Input: part model. Units: mm. Frame: model coordinates. Round coordinates to 2 decimals unless told otherwise and drop trailing zeros. Loops run counter-clockwise (first coordinate to the right, second up) from the corner with the lowest first, then second, coordinate; pieces in that order, holes last.
(1) First-contact query: pin 1 Ø2.5 at (x, y) = (12, -35) entering from +Z. Flat tip, straight axial feed; report the tip coordinate or a pass-through.
(2) Line query: line 1 (X direction, y = -12, z = 1.5); line 2 (Y direction, x = 31, z = 3); line 3 (X direction, y = -35, z = 3.5). Output: solid intervals per line, ascending.
(3) Cut plane D-D, the plane z = 3.25. Give the number of separate pieces and of enclosed holes in the cut face, and give its area (3 significant figures).
(4) Cut plane A-A, the plane x = 77. Output: boundary loops of the cut face in (y, z).
(5) Cut plane C-C, the plane x = 5. Output: boundary loops of the cut face in (y, z), and give its area (3 significant figures).
(6) Cut plane B-B, the plane y = -20.5. Output: boundary loops of the cut face in (x, z), and give its area (3 significant figures).
from build123d import *

# Parameters (mm, degrees)
F0_W     = 100
F0_H     = 40
F1_DEPTH = 5
F2_R     = 2.25
F3_DEPTH = 18.9
F5_DEPTH = 0.5
F7_DEPTH = 5


with BuildPart() as f1:
    # F0 (on Top) → F1 (new body)
    with BuildSketch(Plane.XY):
        with Locations((50, -20)):
            Rectangle(F0_W, F0_H)
    extrude(amount=F1_DEPTH)

    # F2 (on Top) → F3 (cut)
    with BuildSketch(Plane.XY):
        with Locations((12, -35)):
            Circle(F2_R)
        with Locations((31, -35)):
            Circle(F2_R)
        with Locations((50, -35)):
            Circle(F2_R)
        with Locations((69, -35)):
            Circle(F2_R)
        with Locations((88, -35)):
            Circle(F2_R)
        with Locations((95, -28)):
            Circle(F2_R)
        with Locations((95, -12)):
            Circle(F2_R)
        with Locations((88, -5)):
            Circle(F2_R)
        with Locations((69, -5)):
            Circle(F2_R)
        with Locations((50, -5)):
            Circle(F2_R)
        with Locations((31, -5)):
            Circle(F2_R)
        with Locations((12, -5)):
            Circle(F2_R)
        with Locations((5, -12)):
            Circle(F2_R)
        with Locations((5, -28)):
            Circle(F2_R)
    extrude(amount=F3_DEPTH, mode=Mode.SUBTRACT)

    # F4 (on face) → F5 (cut)
    with BuildSketch(Plane(origin=(0, 0, 0), x_dir=(1, 0, 0), z_dir=(0, 0, -1))):
        with BuildLine():
            ThreePointArc((91.5, 26.5), (90.972136, 28.736068), (89.5, 30.5))
            ThreePointArc((89.5, 30.5), (88.081139, 31.243416), (86.5, 31.5))
            Line((86.5, 31.5), (13.5, 31.5))
            ThreePointArc((13.5, 31.5), (9.964466, 30.035534), (8.5, 26.5))
            Line((8.5, 26.5), (8.5, 13.5))
            ThreePointArc((8.5, 13.5), (9.964466, 9.964466), (13.5, 8.5))
            Line((13.5, 8.5), (86.5, 8.5))
            ThreePointArc((86.5, 8.5), (90.035534, 9.964466), (91.5, 13.5))
            Line((91.5, 13.5), (91.5, 26.5))
        make_face()
        with BuildLine():
            ThreePointArc((10.5, 26.5), (11.37868, 28.62132), (13.5, 29.5))
            Line((13.5, 29.5), (86.5, 29.5))
            ThreePointArc((86.5, 29.5), (88.62132, 28.62132), (89.5, 26.5))
            Line((89.5, 26.5), (89.5, 13.5))
            ThreePointArc((89.5, 13.5), (88.62132, 11.37868), (86.5, 10.5))
            Line((86.5, 10.5), (13.5, 10.5))
            ThreePointArc((13.5, 10.5), (11.37868, 11.37868), (10.5, 13.5))
            Line((10.5, 13.5), (10.5, 26.5))
        make_face(mode=Mode.SUBTRACT)
    extrude(amount=-F5_DEPTH, mode=Mode.SUBTRACT)

    # F6 (on face) → F7 (cut)
    with BuildSketch(Plane(origin=(0, 0, 0), x_dir=(1, 0, 0), z_dir=(0, 0, -1))):
        Polygon((85, 13.5), (86.5, 13.5), (86.5, 26.5), (73.5, 26.5), (73.5, 13.5), (84, 13.5), align=None)
        Polygon((26.5, 13.5), (26.5, 26.5), (13.5, 26.5), (13.5, 13.5), (16, 13.5), align=None)
    extrude(amount=-F7_DEPTH, mode=Mode.SUBTRACT)


solid = f1.part
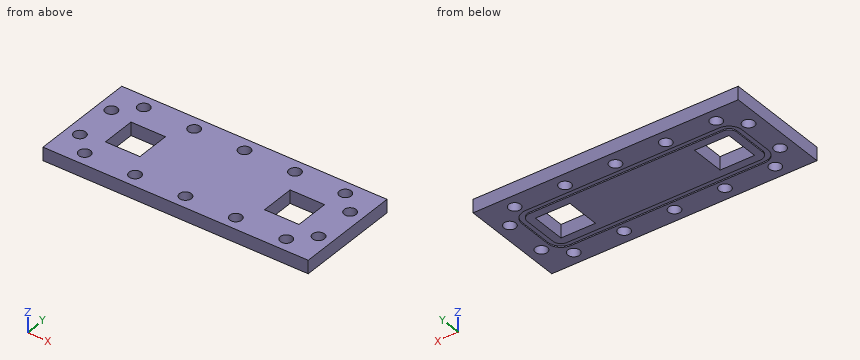
Reported:
1. pin 1: passes through
2. line 1: x = 0 to 2.75, 7.25 to 92.75, 97.25 to 100
2. line 2: y = -40 to -37.25, -32.75 to -7.25, -2.75 to 0
2. line 3: x = 0 to 9.75, 14.25 to 28.75, 33.25 to 47.75, 52.25 to 66.75, 71.25 to 85.75, 90.25 to 100
3. separate pieces: 1
3. enclosed holes: 16
3. area: 3,440 mm2
4. outline: (-40, 0) - (-31.5, 0) - (-31.5, 0.5) - (-29.5, 0.5) - (-29.5, 0) - (-26.5, 0) - (-26.5, 5) - (-40, 5) - close; (-13.5, 0) - (-10.5, 0) - (-10.5, 0.5) - (-8.5, 0.5) - (-8.5, 0) - (0, 0) - (0, 5) - (-13.5, 5) - close
5. outline: (-40, 0) - (-30.25, 0) - (-30.25, 5) - (-40, 5) - close; (-25.75, 0) - (-14.25, 0) - (-14.25, 5) - (-25.75, 5) - close; (-9.75, 0) - (0, 0) - (0, 5) - (-9.75, 5) - close
5. area: 155 mm2
6. outline: (0, 0) - (8.5, 0) - (8.5, 0.5) - (10.5, 0.5) - (10.5, 0) - (13.5, 0) - (13.5, 5) - (0, 5) - close; (26.5, 0) - (73.5, 0) - (73.5, 5) - (26.5, 5) - close; (86.5, 0) - (89.5, 0) - (89.5, 0.5) - (91.5, 0.5) - (91.5, 0) - (100, 0) - (100, 5) - (86.5, 5) - close
6. area: 368 mm2
